Autodesk Inventor part; units mm, degrees
ref_plane "Work Plane1" through (87.1212, -240.6892, 0) normal (1, 0, 0) x (0, 0, -1)
ref_plane "YZ Plane" through (0, 0, 0) normal (1, 0, 0) x (0, 1, 0)
ref_plane "XZ Plane" through (0, 0, 0) normal (0, 1, 0) x (-1, 0, 0)
sketch "Sketch1" plane through (0, 0, 0) normal (0, 0, 1) x (1, 0, 0)
  line L0 (-14.4788, 22.2008) -> (188.7212, 22.2008)
  line L1 (188.7212, 22.2008) -> (188.7212, -240.6892)
  line L2 (188.7212, -240.6892) -> (-14.4788, -240.6892)
  line L3 (-14.4788, -240.6892) -> (-14.4788, 22.2008)
  dimension "d0" = 203.2
  dimension "d1" = 262.89
extrude "Extrusion1" add sketch "Sketch1" along normal blind 38.1
sketch "Sketch2" plane through (0, 0, 38.1) normal (0, 0, 1) x (1, 0, 0)
  line L0 (188.7212, 22.2008) -> (188.7212, -240.6892)
  line L1 (-14.4788, 22.2008) -> (188.7212, 22.2008)
  point P0 (87.1212, -109.2442)
  dimension "d4" = 101.6
  dimension "d5" = 131.445
hole "Hole1" at (87.1212, -109.2442, 38.1) direction (0, 0, -1) diameter 13.3858 end through all
sketch "Sketch3" plane through (0, 0, 38.1) normal (0, 0, 1) x (1, 0, 0)
  circle A0 centre (87.1212, -109.2442) radius 6.6929
  point P0 (87.1212, 3.2016)
  point P1 (87.1212, -221.69)
  dimension "d13" = 112.4458
  dimension "d14" = 112.4458
hole "Hole2" at (87.1212, 3.2016, 38.1) at (87.1212, -221.69, 38.1) direction (0, 0, -1) diameter 13.3858 end through all
ref_plane "Work Plane1" through (87.1212, -240.6892, 0) normal (1, 0, 0) x (0, 0, -1)
properties part number "Sideplate"
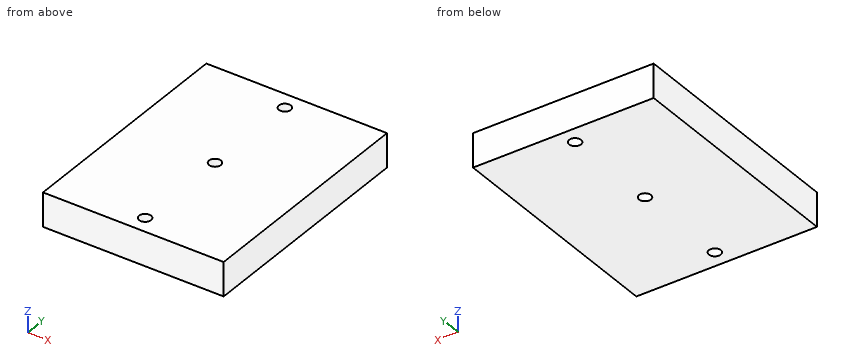
Source: CAD feature listing. Evaluate the final solid. Frame: model axes, mm. Give positions to 0.01 mm unless a question says otherwise; leave off trailing zeros. Write each loop counter-clockwise with the first axis right and the second up, starting at its lowest first coordinate (ties: lowest second). Pieces come first, ordered by that corner, then holes. Notation, with made-up numbers: (-3, 17.5) - (55, 17.5) arc R9 cw to (55, 32.5) - close; hole circle Ø8 at (-4.75, 7.5). An arc over 180 degrees is marked (long way). Write item = value, one per line. Start each with the question number.
Q1. Pin query (flat end, axial travel): pin 1 Ø8 at (x, y) = (87.12, 3.2) entering from -Z; pin 2 Ø3 at (x, y) = (63, -112.5) entering from -Z. Return the tip coordinate at first contact, or that it passes through.
Q2. Material intervals for probe 1 along X at (y, z) = (-221.69, 27); probe 2 along X at (y, z) = (-221, 26); probe 3 along Y at (x, z) = (91, 20), sorted ascending.
Q3. Cut plane A-A, the plane y = -221.69. Return loops of the section in (x, z), then the cut area to 3 significant figures.
Computed values:
q1.pin_1 = through
q1.pin_2 = 0
q2.probe_1 = -14.48 to 80.43, 93.81 to 188.72
q2.probe_2 = -14.48 to 80.46, 93.78 to 188.72
q2.probe_3 = -240.69 to -227.14, -216.24 to -114.7, -103.79 to -2.25, 8.66 to 22.2
q3.outline = (-14.48, 0) - (80.43, 0) - (80.43, 38.1) - (-14.48, 38.1) - close; (93.81, 0) - (188.72, 0) - (188.72, 38.1) - (93.81, 38.1) - close
q3.area = 7,230 mm²
